Print and shaded views of the part. All mm, measured from the part's lowest x, y and z. Give positions to 0.01 mm unless a question says otherwise; leave off trailing zeros. Loops run counter-clockwise (first coordinate to the right, second up) from the corner with the lowest first, then second, coordinate; pieces in that order, holes last.
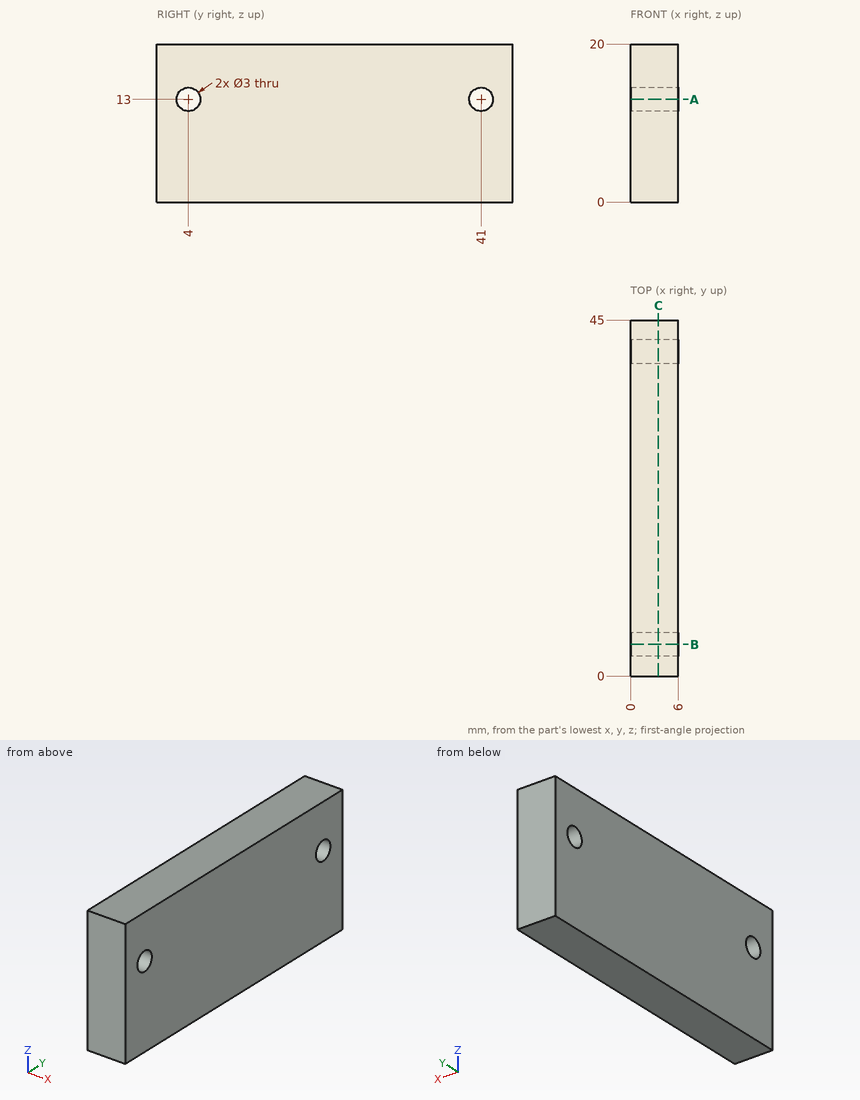
1. Probe line 1 along Y through (x, z) = (1.65, 13); line 2 along Z through (x, y) = (5.55, 40.5). List the from-to ranges inside material, lowest first.
Responses:
line 1: y = 0 to 2.5, 5.5 to 39.5, 42.5 to 45
line 2: z = 0 to 11.59, 14.41 to 20
2. Drop a flat-ended pin along its axis: pin 1 (2.5 mm diameter, centred on y = 4, z = 13, fed in from +X) (3 decimals). Give the stop position or say it passes through.
Responses:
pin 1: passes through
3. Saw through at A-A, the plane z = 13. List the corners of the cut face in (x, y), and give its area (3 significant figures).
Responses:
outline: (0, 0) - (6, 0) - (6, 2.5) - (0, 2.5) - close; (0, 5.5) - (6, 5.5) - (6, 39.5) - (0, 39.5) - close; (0, 42.5) - (6, 42.5) - (6, 45) - (0, 45) - close
area: 234 mm2
4. Saw through at B-B, the plane y = 4. List the corners of the cut face in (x, z), and give its area (3 significant figures).
Responses:
outline: (0, 0) - (6, 0) - (6, 11.5) - (0, 11.5) - close; (0, 14.5) - (6, 14.5) - (6, 20) - (0, 20) - close
area: 102 mm2
5. Saw through at C-C, the plane x = 3.5. List the corners of the cut face in (y, z).
Responses:
outline: (0, 0) - (45, 0) - (45, 20) - (0, 20) - close; hole circle Ø3 at (4, 13); hole circle Ø3 at (41, 13)
